```python
from build123d import *

# Parameters (mm, degrees)
BOSS_EXTRUDE2_DEPTH      = 3.5
BOSS_EXTRUDE2_DEPTH_BACK = 1.5
SKETCH2_W                = 34.5
SKETCH2_H                = 14
SKETCH2_W_2              = 2.5
SKETCH2_H_2              = 10
SKETCH2_W_3              = 26
BOSS_EXTRUDE5_DEPTH      = 3.5
BOSS_EXTRUDE5_DEPTH_BACK = 4.5
SKETCH9_W                = 30.5
SKETCH9_H                = 16
CUT_EXTRUDE1_DEPTH       = 2
CUT_EXTRUDE2_DEPTH       = 8
BOSS_EXTRUDE4_DEPTH      = 3
SKETCH5_W                = 7
SKETCH5_H                = 1
CUT_EXTRUDE3_DEPTH       = 1
CUT_EXTRUDE4_DEPTH       = 6
CUT_EXTRUDE4_DEPTH_BACK  = 6
SKETCH7_R                = 0.2


with BuildPart() as part:
    # Sketch2 → Boss-Extrude2 (new, two sides: drawn at the far end of the back side and taken through both)
    with BuildSketch(Plane(origin=(0, 0, 0), x_dir=(1, 0, 0), z_dir=(0, 1, 0)).offset(-BOSS_EXTRUDE2_DEPTH_BACK)):
        Rectangle(SKETCH2_W, SKETCH2_H)
        with Locations((-14, 0)):
            Rectangle(SKETCH2_W_2, SKETCH2_H_2, mode=Mode.SUBTRACT)
        with Locations((2.25, 0)):
            Rectangle(SKETCH2_W_3, SKETCH2_H_2, mode=Mode.SUBTRACT)
    extrude(amount=BOSS_EXTRUDE2_DEPTH + BOSS_EXTRUDE2_DEPTH_BACK)

    # Sketch9 → Boss-Extrude5 (add, two sides: drawn at the far end of the back side and taken through both)
    with BuildSketch(Plane(origin=(0, 0, 0), x_dir=(1, 0, 0), z_dir=(0, 1, 0)).offset(-BOSS_EXTRUDE5_DEPTH_BACK)):
        Polygon((17.25, -10), (17.25, 8), (17.25, 10), (15.25, 10), (-15.25, 10), (-17.25, 10), (-17.25, 8), (-17.25, -10), align=None)
        Rectangle(SKETCH9_W, SKETCH9_H, mode=Mode.SUBTRACT)
    extrude(amount=BOSS_EXTRUDE5_DEPTH + BOSS_EXTRUDE5_DEPTH_BACK)

    # Sketch3 → Cut-Extrude1 (cut)
    with BuildSketch(Plane(origin=(17.25, 0, 0), x_dir=(0, 0, -1), z_dir=(1, 0, 0))):
        Polygon((-1.5, 0), (-1.5, 3.1), (1.5, 3.1), (1.5, 0), (1.5, -0.1), (-1.5, -0.1), align=None)
    extrude(amount=-CUT_EXTRUDE1_DEPTH, mode=Mode.SUBTRACT)

    # Sketch4 → Cut-Extrude2 (cut)
    with BuildSketch(Plane.ZY.offset(17.25)):
        Polygon((-1.5, -0.1), (1.5, -0.1), (1.5, 0), (1.5, 3.1), (-1.5, 3.1), (-1.5, 0), align=None)
    extrude(amount=-CUT_EXTRUDE2_DEPTH, mode=Mode.SUBTRACT)

    # Sketch1 → Boss-Extrude4 (add)
    with BuildSketch(Plane(origin=(0, 0, 0), x_dir=(1, 0, 0), z_dir=(0, 1, 0))):
        Polygon((-1.07297499, -1.25), (4.486628642, -5), (4.486628642, -6), (6.049148178, -6), (6.049148178, -5), (0.35765833, -1.25), (1.07297499, -1.25), (23.92702501, -1.25), (23.92702501, 1.25), (1.07297499, 1.25), (0.35765833, 1.25), (6.049148178, 5), (6.049148178, 6), (4.486628642, 6), (4.486628642, 5), (-1.07297499, 1.25), align=None)
    extrude(amount=BOSS_EXTRUDE4_DEPTH)

    # Sketch5 → Cut-Extrude3 (cut)
    with BuildSketch(Plane.XZ):
        with Locations((3.5, 0)):
            Rectangle(SKETCH5_W, SKETCH5_H)
    extrude(amount=-CUT_EXTRUDE3_DEPTH, mode=Mode.SUBTRACT)

    # Sketch7 → Cut-Extrude4 (cut, two sides: drawn at the far end of the back side and taken through both)
    with BuildSketch(Plane.XY.offset(-CUT_EXTRUDE4_DEPTH_BACK)):
        with Locations((3.5, -1.2)):
            Circle(SKETCH7_R)
    extrude(amount=CUT_EXTRUDE4_DEPTH + CUT_EXTRUDE4_DEPTH_BACK, mode=Mode.SUBTRACT)


solid = part.part
```
Work out the finished part from the listing and answer in its coordinate system (mm). A direction names the side the tool comes from. Give positions to 0.01 mm unless a question says otherwise; leave off trailing zeros. Write each loop counter-clockwise with the first axis right and the second up, starting at its lowest first coordinate (ties: lowest second). Pieces come first, ordered by that corner, then holes. Notation, with made-up numbers: (60.5, 34.5) -> (114.5, 34.5) arc R10 cw to (114.5, 46.5) -> close; hole circle Ø4 at (83.25, -10.5). An arc over 180 degrees is marked (long way). Write each question's results on one line, items separated by ' | '.
1. Find section B-B on x = -3. Determine the outline of the cut face in (y, z).
Data:
outline: (-4.5, -10) -> (3.5, -10) -> (3.5, -8) -> (-4.5, -8) -> close; (-4.5, 8) -> (3.5, 8) -> (3.5, 10) -> (-4.5, 10) -> close; (-1.5, -7) -> (3.5, -7) -> (3.5, -5) -> (-1.5, -5) -> close; (-1.5, 5) -> (3.5, 5) -> (3.5, 7) -> (-1.5, 7) -> close
2. A tool of negligible diameter and unlimited length cuts with its end or side. For faces 1 (the flat face through (-12, 1, 1.5)), 2 (the flat face through (7, 0.5, 0)), 3 (the flat face through (-12, 3.1, 0)), 4 (the flat face through (-0.1, -4.5, -8.2)), 5 (the flat face through (3.24, 1.48, 3.15)), from which of +Z, -Z, +X, -X, +Y, -Y can it reach the whole face along a straight path? Write none if from no direction.
Data:
face 1: -X | face 2: -Y | face 3: +X, -X | face 4: +Z, -Z, +X, -X, -Y | face 5: +Y, -Y
3. Determine the mould class of faces 6 (the flat face through (-14, 1, 5)), 7 (the flat face through (0, -1, 10)), 8 (the flat face through (-17.25, -1, 0)), 9 (the flat face through (10, 0, 0)) for opening direction Z: +Z half, -Z half, draft (parallel to the pull), parting line (faces both ways), or undercut.
Data:
face 6: undercut | face 7: +Z half | face 8: draft | face 9: undercut
4. Straight lines are drawn through the part: L1, parallel to X at y = -0.25, z = -3.25; L2, parallel to Z at x = -5, y = -0.5; L3, parallel to Z at x = 17, y = 0.5. For each, find the intervals that lie inside material, in ascending order.
Data:
L1: -17.25 to -15.25, -12.75 to -10.75, 15.25 to 17.25 | L2: -10 to -8, -7 to -5, 5 to 7, 8 to 10 | L3: -10 to -1.5, -1.25 to 1.25, 1.5 to 10
5. Find section A-A on x = -12. Determine the outline of the cut face in (y, z).
Data:
outline: (-4.5, -10) -> (3.5, -10) -> (3.5, -8) -> (-4.5, -8) -> close; (-4.5, 8) -> (3.5, 8) -> (3.5, 10) -> (-4.5, 10) -> close; (-1.5, -7) -> (3.5, -7) -> (3.5, 7) -> (-1.5, 7) -> close; hole (-0.1, -1.5) -> (3.1, -1.5) -> (3.1, 1.5) -> (-0.1, 1.5) -> close
6. Find section D-D on z = -7.5. Determine the outline of the cut face in (x, y), and give its area (3 significant figures).
Data:
outline: (-17.25, -4.5) -> (-15.25, -4.5) -> (-15.25, 3.5) -> (-17.25, 3.5) -> close; (15.25, -4.5) -> (17.25, -4.5) -> (17.25, 3.5) -> (15.25, 3.5) -> close | area: 32.0 mm^2
7. Each of these flat-tipped pins is pushed along its axis until it touches: pin 1 Ø7 at (x, z) = (2.5, 0) entering from -Y; pin 2 Ø2 at (x, z) = (-12, 0) entering from -Y. Where does it stop, or does it pass through?
Data:
pin 1: y = 0 | pin 2: y = -1.5
8. Find section C-C on y = -3.5. Determine the outline of the cut face in (x, z), and give its area (3 significant figures).
Data:
outline: (-17.25, -10) -> (17.25, -10) -> (17.25, 10) -> (-17.25, 10) -> close; hole (-15.25, -8) -> (15.25, -8) -> (15.25, 8) -> (-15.25, 8) -> close | area: 202 mm^2
